Input: part model. Units: mm. Frame: model coordinates. Face numbers are marked on the shaded views. A direction names the side the tool comes from. Coordinates: 2 decimals unless noted, no trailing zeros. Write each loop counter-clockwise with the first axis right and the second up, starting at its lowest first coordinate (ties: lowest second). Pieces come first, ordered by that corner, then holes. Notation, with made-up numbers: M 44,-32 L 93,-32 A14 ccw 93,-13 Z; hole C 60,53.25 d11. An arc over 180 degrees is marked long. Write each question's results on one line, items separated by ' | '. Start each with the question number.
1. Ray query, probe 1 along Y at (x, z) = (9.25, -0.5); probe 2 along Z at (x, y) = (13, 8); probe 3 along Y at (x, z) = (-2, -2). Return the intervals inside material, ascending.
2. Section query D-D, the plane z = -5. Output: boundary loops of the cut face in (x, y), and give its area (3 significant figures).
3. Section query A-A, the plane y = 51. Output: boundary loops of the cut face in (x, z).
4. Pull-direction query (X, two-part tool) for the marked faces 6, 7 and 8; classes: +X half, -X half, draft (parallel to the pull), parting line (faces both ways), or undercut.
5. Set-up query: the marked faces 1, 2, 3, 4 and 5. Return all of +Z, -Z, +X, -X, +Y, -Y with unobstructed straight access to the full face (end or side cutting, diameter ignored); none if empty.
6. First-contact query: pin 1 (4 mm diameter, centred on x = 3, z = -58.5, fed in from +Y); pin 2 (7 mm diameter, centred on x = 0, z = -35.5, fed in from -Y); pin 3 (6 mm diameter, centred on y = 46, z = -45.5, fed in from +X). Flat tips, straight axial feed; report the tip coordinate or a pass-through.
```python
from build123d import *

# Parameters (mm, degrees)
SKETCH_14_W          = 13.892097438
SKETCH_14_H          = 8.107274344
EXTRUDE_7_DEPTH      = 75
EXTRUDE_15_DEPTH     = 12
SKETCH_21_R          = 17
SKETCH_21_R_2        = 14.25
EXTRUDE_16_DEPTH     = 6
EXTRUDE_17_DEPTH     = 6
CUT_EXTRUDE_3_DEPTH  = 6
EXTRUDE_START        = 10
EXTRUDE_18_DEPTH     = 10
SKETCH_26_R          = 2
CUT_EXTRUDE_5_DEPTH  = 102.624375612
SKETCH_27_W          = 25
SKETCH_27_H          = 59
SKETCH_27_R          = 1.75
SKETCH_27_R_2        = 1.5
SKETCH_27_W_2        = 20
SKETCH_27_H_2        = 41
EXTRUDE_20_DEPTH     = 12
SKETCH_29_W          = 25
SKETCH_29_H          = 12
EXTRUDE_21_DEPTH     = 2
SKETCH_31_W          = 13.892097438
SKETCH_31_H          = 75
EXTRUDE_22_DEPTH     = 3.1
SKETCH_33_W          = 25
SKETCH_33_H          = 12
CUT_EXTRUDE_8_DEPTH  = 3.1
CUT_EXTRUDE_START    = -7
SKETCH_34_R          = 1.5
CUT_EXTRUDE_9_DEPTH  = 7
SKETCH_35_W          = 2.5
SKETCH_35_H          = 2
CUT_EXTRUDE_10_DEPTH = 5


with BuildPart() as part:
    # 草圖14 → 填料-伸長7 (new body)
    with BuildSketch(Plane(origin=(0, 0, -8), x_dir=(-1, 0, 0), z_dir=(0, 0, -1))):
        with Locations((-2.293750102, 52.915857713)):
            Rectangle(SKETCH_14_W, SKETCH_14_H)
    extrude(amount=EXTRUDE_7_DEPTH)

    # 草圖15 → 填料-伸長15 (add)
    with BuildSketch(Plane.XZ.offset(-48.862220541)):
        Polygon((2.293750102, -83), (-4.652298617, -83), (-4.652298617, -77), (2.293750102, -77), (9.239798821, -77), (9.239798821, -83), align=None)
    extrude(amount=EXTRUDE_15_DEPTH)

    # 草圖21 → 填料-伸長16 (add)
    with BuildSketch(Plane.XY.offset(-77)):
        with Locations((2.293750102, 22.612220541)):
            Circle(SKETCH_21_R)
        with Locations((2.293750102, 22.612220541)):
            Circle(SKETCH_21_R_2, mode=Mode.SUBTRACT)
    extrude(amount=-EXTRUDE_16_DEPTH)

    # 草圖22 → 填料-伸長17 (add)
    with BuildSketch(Plane.XY.offset(-77)):
        with BuildLine():
            Line((-4.652298617, 7.096022321), (-4.652298617, -0.903977679))
            Line((-4.652298617, -0.903977679), (9.239798821, -0.903977679))
            Line((9.239798821, -0.903977679), (9.239798821, 7.096022321))
            ThreePointArc((9.239798821, 7.096022321), (2.293750102, 5.612220541), (-4.652298617, 7.096022321))
        make_face()
    extrude(amount=-EXTRUDE_17_DEPTH)

    # 草圖23 → 除料-伸長3 (cut)
    with BuildSketch(Plane.XY.offset(-77)):
        with BuildLine():
            Line((2.293750102, 48.862220541), (2.293750102, 36.862220541))
            ThreePointArc((2.293750102, 36.862220541), (-11.956249898, 22.612220541), (2.293750102, 8.362220541))
            Line((2.293750102, 8.362220541), (2.293750102, -0.903977679))
            Line((2.293750102, -0.903977679), (-4.652298617, -0.903977679))
            Line((-4.652298617, -0.903977679), (-4.652298617, 7.096022321))
            ThreePointArc((-4.652298617, 7.096022321), (-14.706249898, 22.612220541), (-4.652298617, 38.12841876))
            Line((-4.652298617, 38.12841876), (-4.652298617, 48.862220541))
            Line((-4.652298617, 48.862220541), (2.293750102, 48.862220541))
        make_face()
    extrude(amount=-CUT_EXTRUDE_3_DEPTH, mode=Mode.SUBTRACT)

    # 草圖25 → 填料-伸長18 (add)
    with BuildSketch(Plane.XY.offset(-77).offset(EXTRUDE_START)):
        with BuildLine():
            Line((2.293750102, -0.903977679), (9.239798821, -0.903977679))
            Line((9.239798821, -0.903977679), (9.239798821, 7.096022321))
            ThreePointArc((9.239798821, 7.096022321), (19.293750102, 22.612220541), (9.239798821, 38.12841876))
            Line((9.239798821, 38.12841876), (9.239798821, 48.862220541))
            Line((9.239798821, 48.862220541), (2.293750102, 48.862220541))
            Line((2.293750102, 48.862220541), (2.293750102, 36.862220541))
            ThreePointArc((2.293750102, 36.862220541), (16.543750102, 22.612220541), (2.293750102, 8.362220541))
            Line((2.293750102, 8.362220541), (2.293750102, -0.903977679))
        make_face()
    extrude(amount=-EXTRUDE_18_DEPTH)

    # 草圖26 → 除料-伸長5 (cut, through all)
    with BuildSketch(Plane(origin=(9.239798821, 0, 0), x_dir=(0, 0, -1), z_dir=(1, 0, 0))):
        with Locations((74.853766884, 3.096022321)):
            Circle(SKETCH_26_R)
        with Locations((74.853766884, 43.49531965)):
            Circle(SKETCH_26_R)
    extrude(amount=-CUT_EXTRUDE_5_DEPTH, mode=Mode.SUBTRACT)

    # 草圖27 → 填料-伸長20 (add)
    with BuildSketch(Plane.XY.offset(-8)):
        with Locations((2.293750102, 28.596022321)):
            Rectangle(SKETCH_27_W, SKETCH_27_H)
        with Locations((-2.356249898, 6.596022321)):
            Circle(SKETCH_27_R, mode=Mode.SUBTRACT)
        with Locations((6.943750102, 6.596022321)):
            Circle(SKETCH_27_R, mode=Mode.SUBTRACT)
        with Locations(Location((-2.356249898, 55.896022321, 0), (0, 0, 134.303638859))):
            Circle(SKETCH_27_R_2, mode=Mode.SUBTRACT)
        with Locations(Location((6.943750102, 55.896022321, 0), (0, 0, 134.303638859))):
            Circle(SKETCH_27_R_2, mode=Mode.SUBTRACT)
        with Locations((2.293750102, 31.396022321)):
            Rectangle(SKETCH_27_W_2, SKETCH_27_H_2, mode=Mode.SUBTRACT)
    extrude(amount=EXTRUDE_20_DEPTH)

    # 草圖29 → 填料-伸長21 (add)
    with BuildSketch(Plane(origin=(0, 58.096022321, 0), x_dir=(1, 0, 0), z_dir=(0, 1, 0))):
        with Locations((2.293750102, 2)):
            Rectangle(SKETCH_29_W, SKETCH_29_H)
    extrude(amount=EXTRUDE_21_DEPTH)

    # 草圖31 → 填料-伸長22 (add)
    with BuildSketch(Plane(origin=(0, 56.969494885, 0), x_dir=(1, 0, 0), z_dir=(0, 1, 0))):
        with Locations((2.293750102, 45.5)):
            Rectangle(SKETCH_31_W, SKETCH_31_H)
    extrude(amount=EXTRUDE_22_DEPTH)

    # 草圖33 → 除料-伸長8 (cut)
    with BuildSketch(Plane.XZ.offset(0.903977679)):
        with Locations((2.293750102, -2)):
            Rectangle(SKETCH_33_W, SKETCH_33_H)
    extrude(amount=-CUT_EXTRUDE_8_DEPTH, mode=Mode.SUBTRACT)

    # 草圖34 → 除料-伸長9 (cut)
    with BuildSketch(Plane.XY.offset(-8).offset(CUT_EXTRUDE_START)):
        with Locations((6.943750102, 55.896022321)):
            Circle(SKETCH_34_R)
        with Locations((-2.356249898, 55.896022321)):
            Circle(SKETCH_34_R)
    extrude(amount=CUT_EXTRUDE_9_DEPTH, mode=Mode.SUBTRACT)

    # 草圖35 → 除料-伸長10 (cut)
    with BuildSketch(Plane.XY.offset(4)):
        with Locations((2.293750102, 52.896022321)):
            Rectangle(SKETCH_35_W, SKETCH_35_H)
        with Locations((2.293750102, 9.896022321)):
            Rectangle(SKETCH_35_W, SKETCH_35_H)
    extrude(amount=-CUT_EXTRUDE_10_DEPTH, mode=Mode.SUBTRACT)


solid = part.part
```
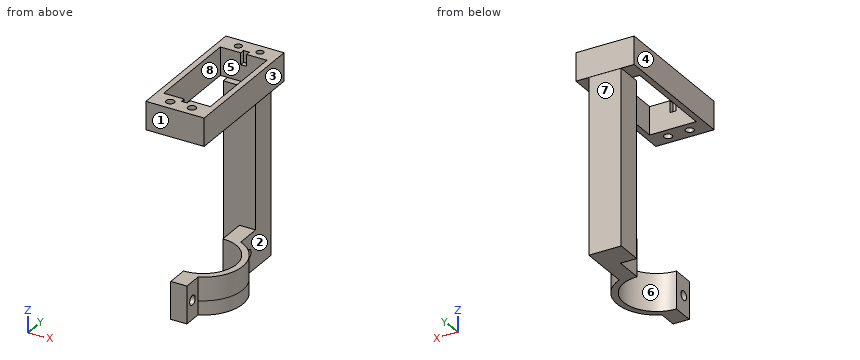
Answer:
1) probe 1: 2.2 to 10.9, 51.9 to 60.1 | probe 2: -8 to 4 | probe 3: 2.2 to 4.88, 8.31 to 10.9, 51.9 to 54.44, 57.35 to 60.1
2) outline: M -10.21,2.2 L 14.79,2.2 L 14.79,60.1 L -10.21,60.1 Z; hole M -7.71,10.9 L 12.29,10.9 L 12.29,51.9 L -7.71,51.9 Z; hole C -2.36,6.6 d3.5; hole C -2.36,55.9 d3; hole C 6.94,6.6 d3.5; hole C 6.94,55.9 d3 | area: 594 mm^2
3) outline: M -10.21,-8 L -7.71,-8 L -7.71,4 L -10.21,4 Z; M -4.65,-83 L 9.24,-83 L 9.24,-8 L -4.65,-8 Z; M 12.29,-8 L 14.79,-8 L 14.79,4 L 12.29,4 Z
4) face 6: -X half | face 7: draft | face 8: undercut
5) face 1: +Z, +X, -X, -Y | face 2: -Z, +X, +Y | face 3: +Z, +X, +Y, -Y | face 4: +Z, -Z, -X, +Y, -Y | face 5: +Z
6) pin 1: y = 60.07 | pin 2: y = 48.86 | pin 3: x = 9.24
